Read the model definition and answer for the solid it produces. Units are mm, in the model's axes. A direction names the side the tool comes from. Round coordinates to 2 decimals unless told otherwise and drop trailing zeros. Write each loop counter-clockwise with the first axis right and the second up, starting at its lowest first coordinate (ties: lowest second). Pieces come first, ordered by that corner, then holes. Notation, with made-up numbers: (-31.75, 45.5) -> (-20.75, 45.5) arc R16 ccw to (-20.75, 66.5) -> close; hole circle Ø10 at (-15.75, -13.75). An arc over 180 degrees is marked (long way). Return JSON: item names as keys, results as strings.
from build123d import *

# Parameters (mm, degrees)
F0_W     = 55
F0_H     = 100
F1_DEPTH = 1.5
F2_R     = 3
F3_R     = 2.4
F4_DEPTH = 4.5
F5_R     = 1.65
F6_DEPTH = 2


with BuildPart() as f1:
    # F0 (on Top) → F1 (new body)
    with BuildSketch(Plane.XY):
        with Locations((27.5, 50)):
            Rectangle(F0_W, F0_H)
    extrude(amount=F1_DEPTH)

    # F2
    f2_edges = [f1.edges().sort_by_distance(p)[0] for p in [
        (0, 100, 0.75),
        (55, 100, 0.75),
        (0, 0, 0.75),
        (55, 0, 0.75),
    ]]
    fillet(f2_edges, radius=F2_R)

    # F3 (on face) → F4 (join)
    with BuildSketch(Plane.XY.offset(1.5)):
        with Locations((4, 96)):
            Circle(F3_R)
        with Locations((4, 4)):
            Circle(F3_R)
        with Locations((51, 96)):
            Circle(F3_R)
        with Locations((51, 4)):
            Circle(F3_R)
    extrude(amount=F4_DEPTH)

    # F5 (on face) → F6 (cut)
    with BuildSketch(Plane.XY.offset(6)):
        with Locations((4, 96)):
            Circle(F5_R)
        with Locations((4, 4)):
            Circle(F5_R)
        with Locations((51, 96)):
            Circle(F5_R)
        with Locations((51, 4)):
            Circle(F5_R)
    extrude(amount=-F6_DEPTH, mode=Mode.SUBTRACT)


solid = f1.part
Item 1: Section D-D (y = 63) is taken. Give the vertices of the cut face in (x, z), then the cut area to 3 significant figures.
Worked answers:
{"outline": "(0, 0) -> (55, 0) -> (55, 1.5) -> (0, 1.5) -> close", "area": "82.5 mm2"}
Item 2: A tool of negligible diameter and unlimited length cuts with its end or side. For faces 1 (the cylindrical face through (49.35, 4.07, 5.01)), 2 (the flat face through (6, 97, 6)), from which of +Z, -Z, +X, -X, +Y, -Y can it reach the whole face along a straight path? Write none if from no direction.
Worked answers:
{"face 1": "+Z", "face 2": "+Z, +X, -X, +Y, -Y"}
Item 3: Section A-A (y = 4) is taken. Give the vertices of the cut face in (x, z), then the cut area to 4 significant figures.
Worked answers:
{"outline": "(0, 0) -> (55, 0) -> (55, 1.5) -> (53.4, 1.5) -> (53.4, 6) -> (52.65, 6) -> (52.65, 4) -> (49.35, 4) -> (49.35, 6) -> (48.6, 6) -> (48.6, 1.5) -> (6.4, 1.5) -> (6.4, 6) -> (5.65, 6) -> (5.65, 4) -> (2.35, 4) -> (2.35, 6) -> (1.6, 6) -> (1.6, 1.5) -> (0, 1.5) -> close", "area": "112.5 mm2"}
Item 4: Flat-ended cylindrical pins translate along their axes: pin 1 (1.6 mm diameter, centred on x = 51.5, y = 4, fed in from +Z); pin 2 (4 mm diameter, centred on x = 32, y = 13.5, fed in from +Z). Find the tip coordinate at first contact, or state that the pin passes through.
Worked answers:
{"pin 1": "stops at z = 4", "pin 2": "stops at z = 1.5"}
Item 5: Straight lines are drawn through the part: L1, parallel to Y at x = 51, z = 5; L2, parallel to Z at x = 31.5, y = 85. For each, find the intervals that lie inside material, in ascending order. Write a range as [from, to].
Worked answers:
{"L1": "y = [1.6, 2.35], [5.65, 6.4], [93.6, 94.35], [97.65, 98.4]", "L2": "z = [0, 1.5]"}
Item 6: For a pull along Y with two mould halves and no side action, classify faces 3 (the cylindrical face through (2.69, 3, 5.01)), 4 (the cylindrical face through (54.14, 99.1, 0.76)), 5 (the flat face through (50, 94, 6)) as released by +Y, released by -Y, zero draft, split by the parting line, or undercut.
Worked answers:
{"face 3": "undercut", "face 4": "released by +Y", "face 5": "zero draft"}
Item 7: Section B-B (x = 4) is taken. Give the vertices of the cut face in (y, z).
Worked answers:
{"outline": "(0, 0) -> (100, 0) -> (100, 1.5) -> (98.4, 1.5) -> (98.4, 6) -> (97.65, 6) -> (97.65, 4) -> (94.35, 4) -> (94.35, 6) -> (93.6, 6) -> (93.6, 1.5) -> (6.4, 1.5) -> (6.4, 6) -> (5.65, 6) -> (5.65, 4) -> (2.35, 4) -> (2.35, 6) -> (1.6, 6) -> (1.6, 1.5) -> (0, 1.5) -> close"}
Item 8: Section C-C (z = 2.75) is taken. Give the vertices of the cut face in (x, y).
Worked answers:
{"outline": "circle Ø4.8 at (4, 4); circle Ø4.8 at (4, 96); circle Ø4.8 at (51, 4); circle Ø4.8 at (51, 96)"}
